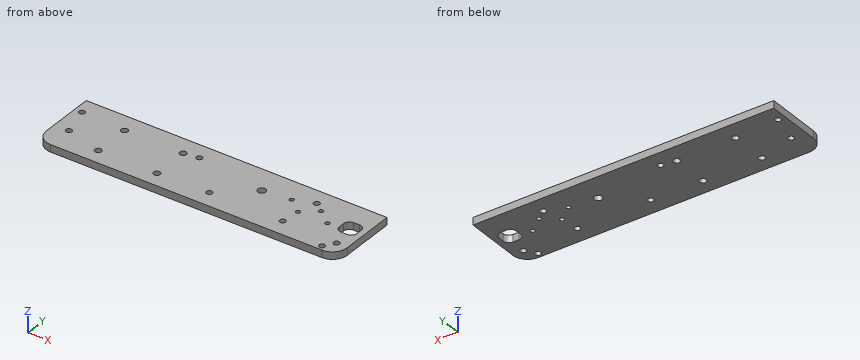
from build123d import *

# Parameters (mm, degrees)
SKETCH_1_R              = 2
EXTRUDE_1_DEPTH         = 5
SKETCH_2_R              = 2.75
SKETCH_2_R_2            = 2
SKETCH_2_R_3            = 2.25
CUT_EXTRUDE_2_DEPTH     = 6
CUT_EXTRUDE_3_OUTLINE_R = 1.5
CUT_EXTRUDE_3_DEPTH     = 5


# Read off the part's stored shape, not the designer's step: 切除-拉伸3
with BuildPart() as part:
    # 草图1 → 凸台-拉伸1 (new body)
    with BuildSketch(Plane.XY):
        with BuildLine():
            Line((-85, 0), (120, 0))
            Line((120, 0), (120, -38))
            ThreePointArc((120, -38), (117.071067812, -45.071067812), (110, -48))
            Line((110, -48), (-75, -48))
            ThreePointArc((-75, -48), (-82.071067812, -45.071067812), (-85, -38))
            Line((-85, -38), (-85, 0))
        make_face()
        with Locations((-80, -11)):
            Circle(SKETCH_1_R, mode=Mode.SUBTRACT)
        with Locations((0, -11)):
            Circle(SKETCH_1_R, mode=Mode.SUBTRACT)
        with Locations((80, -11)):
            Circle(SKETCH_1_R, mode=Mode.SUBTRACT)
        with Locations((75, -36.5)):
            Circle(SKETCH_1_R, mode=Mode.SUBTRACT)
        with Locations(Location((-75, -30.5, 0), (0, 0, 180))):
            Circle(SKETCH_1_R, mode=Mode.SUBTRACT)
        with Locations((25, -36.5)):
            Circle(SKETCH_1_R, mode=Mode.SUBTRACT)
    extrude(amount=EXTRUDE_1_DEPTH)

    # 草图2 → 切除-拉伸2 (cut)
    with BuildSketch(Plane.XY):
        with Locations(Location((47.5, -18, 0), (0, 0, 180))):
            Circle(SKETCH_2_R)
        with Locations(Location((112.5, -37.5, 0), (0, 0, 180))):
            Circle(SKETCH_2_R_2)
        with Locations(Location((107.5, -44.5, 0), (0, 0, 180))):
            Circle(SKETCH_2_R_2)
        with BuildLine():
            ThreePointArc((104, -23), (105.171572875, -25.828427125), (108, -27))
            Line((108, -27), (112, -27))
            ThreePointArc((112, -27), (114.828427125, -25.828427125), (116, -23))
            Line((116, -23), (116, -19))
            ThreePointArc((116, -19), (114.828427125, -16.171572875), (112, -15))
            Line((112, -15), (108, -15))
            ThreePointArc((108, -15), (105.171572875, -16.171572875), (104, -19))
            Line((104, -19), (104, -23))
        make_face()
        with Locations(Location((-50, -12.5, 0), (0, 0, 180))):
            Circle(SKETCH_2_R_3)
        with Locations(Location((-10, -12.5, 0), (0, 0, 180))):
            Circle(SKETCH_2_R_3)
        with Locations(Location((-50, -37.5, 0), (0, 0, 180))):
            Circle(SKETCH_2_R_3)
        with Locations(Location((-10, -37.5, 0), (0, 0, 180))):
            Circle(SKETCH_2_R_3)
    extrude(amount=CUT_EXTRUDE_2_DEPTH, mode=Mode.SUBTRACT)

    # 切除-拉伸3 outline → 切除-拉伸3 (cut)
    with BuildSketch(Plane.XY):
        with Locations((96.5, -24)):
            Circle(CUT_EXTRUDE_3_OUTLINE_R)
        with Locations((86.5, -16)):
            Circle(CUT_EXTRUDE_3_OUTLINE_R)
        with Locations((76.5, -24)):
            Circle(CUT_EXTRUDE_3_OUTLINE_R)
        with Locations((66.5, -16)):
            Circle(CUT_EXTRUDE_3_OUTLINE_R)
    extrude(amount=CUT_EXTRUDE_3_DEPTH, mode=Mode.SUBTRACT)


solid = part.part
Could you check a few things on this model? Use its own coordinates, in mm. Round coordinates to 2 decimals unless told otherwise and drop trailing zeros. Write each loop counter-clockwise with the first axis right and the second up, starting at its lowest first coordinate (ties: lowest second). Pieces come first, ordered by that corner, then holes. Notation, with made-up numbers: (-30, 80) - (-1, 80) arc R11 cw to (-1, 98) - close; hole circle Ø6 at (-19.75, 85.5). An arc over 180 degrees is marked (long way). Use a Markdown table: item, result.
Q1. I want a section at C-C (x = -10). List the corners of the cut face in (y, z) for me, plus the area to 3 significant figures.
Output values:
| item | result |
|---|---|
| outline | (-48, 0) - (-39.75, 0) - (-39.75, 5) - (-48, 5) - close; (-35.25, 0) - (-14.75, 0) - (-14.75, 5) - (-35.25, 5) - close; (-10.25, 0) - (0, 0) - (0, 5) - (-10.25, 5) - close |
| area | 195 mm2 |
Q2. I want a section at A-A (y = -30.5). List the corners of the cut face in (x, z) for me.
Output values:
| item | result |
|---|---|
| outline | (-85, 0) - (-77, 0) - (-77, 5) - (-85, 5) - close; (-73, 0) - (120, 0) - (120, 5) - (-73, 5) - close |
Q3. I want a section at B-B (x = 47.5). List the corners of the cut face in (y, z) for me, plus the area to 4 significant figures.
Output values:
| item | result |
|---|---|
| outline | (-48, 0) - (-20.75, 0) - (-20.75, 5) - (-48, 5) - close; (-15.25, 0) - (0, 0) - (0, 5) - (-15.25, 5) - close |
| area | 212.5 mm2 |
Q4. Please list where these lines run through material, in increasing order: L1, parallel to X at y = -37.5, z = 1; L2, parallel to Y at x = 25, z = 2.4; L3, parallel to X at y = -10.5, z = 0.7.
Output values:
| item | result |
|---|---|
| L1 | -85 to -52.25, -47.75 to -12.25, -7.75 to 23.27, 26.73 to 73.27, 76.73 to 110.5, 114.5 to 120 |
| L2 | -48 to -38.5, -34.5 to 0 |
| L3 | -85 to -81.94, -78.06 to -51.03, -48.97 to -11.03, -8.97 to -1.94, 1.94 to 78.06, 81.94 to 120 |
Q5. I want a section at D-D (z = 2.1). Count the separate pieces of the cut face and the enclosed holes in it, plus the area to 3 significant figures.
Output values:
| item | result |
|---|---|
| separate pieces | 1 |
| enclosed holes | 18 |
| area | 9,450 mm2 |
